```python
from build123d import *

# Parameters (mm, degrees)
SKETCH_2_W               = 80
SKETCH_2_H               = 80
EXTRUDE_1_DEPTH          = 3
SKETCH_3_R               = 1.5
CUT_EXTRUDE_1_DEPTH      = 3
PATTERN_CIRCULAR_1_COUNT = 4
FILLET_1_R               = 4


with BuildPart() as part:
    # Sketch 2 → Extrude 1 (new body)
    with BuildSketch(Plane(origin=(0, 0, 0), x_dir=(1, 0, 0), z_dir=(0, 1, 0))):
        Rectangle(SKETCH_2_W, SKETCH_2_H)
    extrude(amount=EXTRUDE_1_DEPTH)

    # Sketch 3 → Cut-Extrude 1 (cut)
    with BuildSketch(Plane(origin=(0, 0, 0), x_dir=(1, 0, 0), z_dir=(0, 1, 0))):
        with Locations((0, -36)):
            Circle(SKETCH_3_R)
        with Locations((-35.403805922, -35.403805922)):
            Circle(SKETCH_3_R)
    cut_extrude_1 = extrude(amount=CUT_EXTRUDE_1_DEPTH, mode=Mode.SUBTRACT)

    # Pattern Circular 1: Cut-Extrude 1 ×4 about axis
    pattern_circular_1_axis = Axis((0, 0, 0), (0, 1, 0))
    for i in range(1, PATTERN_CIRCULAR_1_COUNT):
        add(cut_extrude_1.rotate(pattern_circular_1_axis, i * 360 / PATTERN_CIRCULAR_1_COUNT), mode=Mode.SUBTRACT)

    # Fillet 1
    fillet_1_edges = [part.edges().sort_by_distance(p)[0] for p in [
        (40, 1.5, 40),
        (-40, 1.5, 40),
        (-40, 1.5, -40),
        (40, 1.5, -40),
    ]]
    fillet(fillet_1_edges, radius=FILLET_1_R)


solid = part.part
```
Geometry: final body of the model. Coordinates: model frame, mm. Coordinates: 2 decimals unless noted, no trailing zeros. Order: outer loops, then holes, each group sorted by start corner. A loop starts at its lowest first (then second) coordinate and runs counter-clockwise, first axis right, second up. Notation, with made-up numbers: M 10,-9.5 L 59,-9.5 A18 cw 59,23.5 Z; hole C -17.75,51 d5. An arc over 180 degrees is marked long. Answer in a Markdown table with one row per item. Add a question column.
Q1. Section query B-B on x = 0. Return the cut outline in (y, z), and give its area (3 significant figures).
Q2. Line query: L1, parallel to X at y = 1.15, z = 0; L2, parallel to Z at x = 36.5, y = 0.3. Output: solid intervals per line, ascending.
Q3. Contact query for flat-ended pins moving along their axis: P1, Ø3.5, axis at x = 36, z = 0, coming from the -Y side; P2, Ø2.5, axis at x = 0, z = -36, coming from the +Y side. Output: stop coordinate, or through.
Q4. Section query A-A on z = 0. Return the cut outline in (x, y).
Q5. Mould query, pull axis Z, two halves, no side actions, for faces 1 (the cylindrical face through (-38.859, 1.521, 38.797)), 2 (the flat face through (40, 1, 1)), 3 (the cylindrical face through (-36.59, 1.48, 36.32)). Classes: released by +Z, released by -Z, zero draft, split by the parting line, or undercut.
Completed:
| question | item | result |
|---|---|---|
| 1 | outline | M 0,-40 L 3,-40 L 3,-37.5 L 0,-37.5 Z; M 0,-34.5 L 3,-34.5 L 3,34.5 L 0,34.5 Z; M 0,37.5 L 3,37.5 L 3,40 L 0,40 Z |
| 1 | area | 222 mm2 |
| 2 | L1 | x = -40 to -37.5, -34.5 to 34.5, 37.5 to 40 |
| 2 | L2 | z = -39.97 to -36.43, -34.38 to -1.41, 1.41 to 34.38, 36.43 to 39.97 |
| 3 | P1 | stops at y = 0 |
| 3 | P2 | passes through |
| 4 | outline | M -40,0 L -37.5,0 L -37.5,3 L -40,3 Z; M -34.5,0 L 34.5,0 L 34.5,3 L -34.5,3 Z; M 37.5,0 L 40,0 L 40,3 L 37.5,3 Z |
| 5 | face 1 | released by +Z |
| 5 | face 2 | zero draft |
| 5 | face 3 | undercut |
